Read the model definition and answer for the solid it produces. Units are mm, in the model's axes. A direction names the side the tool comes from. Coordinates: 2 decimals unless noted, no trailing zeros. Order: outer loops, then holes, each group sorted by start corner. A loop starts at its lowest first (then second) coordinate and runs counter-clockwise, first axis right, second up.
from build123d import *

# Parameters (mm, degrees)
BOSS_EXTRUDE1_DEPTH = 4.7625
SKETCH1_3_W         = 6.35
SKETCH1_3_H         = 9.525
SKETCH1_3_H_2       = 6.35
BOSS_EXTRUDE2_DEPTH = 28.73375
SKETCH2_W           = 12.7
SKETCH2_H           = 6.35
SKETCH2_R           = 2.15265
BOSS_EXTRUDE3_DEPTH = 3.175
FILLET11_R          = 3.81


with BuildPart() as part:
    # Sketch1 → Boss-Extrude1 (new body)
    with BuildSketch(Plane(origin=(0, 0, 0), x_dir=(1, 0, 0), z_dir=(0, 1, 0))):
        Polygon((-49.68875, 4.7625), (-49.68875, -4.7625), (49.68875, -4.7625), (49.68875, 4.7625), (-12.7, 4.7625), (-12.7, 12.303125), (-19.05, 12.303125), (-19.05, 4.7625), align=None)
    extrude(amount=BOSS_EXTRUDE1_DEPTH)

    # Sketch1_3 → Boss-Extrude2 (add)
    with BuildSketch(Plane(origin=(0, 0, 0), x_dir=(1, 0, 0), z_dir=(0, 1, 0))):
        with Locations((-46.51375, 0)):
            Rectangle(SKETCH1_3_W, SKETCH1_3_H)
        with Locations((46.51375, 0)):
            Rectangle(SKETCH1_3_W, SKETCH1_3_H)
        with Locations((-15.875, 9.128125)):
            Rectangle(SKETCH1_3_W, SKETCH1_3_H_2)
    extrude(amount=-BOSS_EXTRUDE2_DEPTH)

    # Mirror1: part across plane


with BuildPart() as part_1:
    add(part.part)
    add(part.part.mirror(Plane(origin=(0, 0, 0), x_dir=(0, 0, 1), z_dir=(1, 0, 0))))

    # Sketch2 → Boss-Extrude3 (add)
    with BuildSketch(Plane.XZ.offset(28.73375)):
        with Locations((-6.35, -9.128125)):
            Rectangle(SKETCH2_W, SKETCH2_H)
        with BuildLine():
            Line((-49.68875, 4.7625), (-49.68875, -13.814359467))
            ThreePointArc((-49.68875, -13.814359467), (-44.838220371, -15.559917245), (-40.842233144, -12.303125))
            Line((-40.842233144, -12.303125), (-15.875, -12.303125))
            Line((-15.875, -12.303125), (-15.875, -5.953125))
            Line((-15.875, -5.953125), (-43.33875, -5.953125))
            Line((-43.33875, -5.953125), (-43.33875, 4.7625))
            Line((-43.33875, 4.7625), (-49.68875, 4.7625))
        make_face()
        with Locations(Location((-45.72, -10.398125, 0), (0, 0, 270))):
            Circle(SKETCH2_R, mode=Mode.SUBTRACT)
    boss_extrude3 = extrude(amount=-BOSS_EXTRUDE3_DEPTH)

    # Mirror3: Boss-Extrude3 across plane
    add(boss_extrude3.mirror(Plane(origin=(0, 0, 0), x_dir=(0, 0, 1), z_dir=(1, 0, 0))))

    # Fillet11
    fillet11_edges = [part_1.edges().sort_by_distance(p)[0] for p in [
        (0, 4.7625, 4.7625),
        (-49.68875, -11.985625, 4.7625),
        (49.68875, -11.985625, 4.7625),
    ]]
    fillet(fillet11_edges, radius=FILLET11_R)


solid = part_1.part
Q1. The part is cut by section C-C, the plane z = -3.5. Determine the outline of the cut face in (x, y), then the cut area to 3 significant figures.
Q2. The part is cut by section B-B, the plane x = 39.5. Determine the outline of the cut face in (y, z), then the cut area to 3 significant figures.
Q3. The part is cut by section A-A, the plane y = -13. Determine the outline of the cut face in (x, z), then the cut area to 3 significant figures.
Q4. Each of these flat-tipped pins is pushed along its axis until it touches: P1, Ø1.4, axis at x = 6.5, y = 3, coming from the -Z side; P2, Ø4, axis at y = -16, z = -10, coming from the +X side; P3, Ø1, axis at x = -33, z = 2, coming from the -Y side; P4, Ø12, axis at x = 35.5, z = -7.5, coming from the +Y side. Where does it stop, or does it pass through?
Q5. Determine the mould class of faces 1 (the cylindrical face through (-48.6, -11.75, 3.62)), 2 (the cylindrical face through (47.82, -27.17, -9.93)), 3 (the flat face through (0, 2, -4.762)), 4 (the cylindrical face through (0.696, 3.617, 3.676)) for opening direction X: +X half, -X half, draft (parallel to the pull), parting line (faces both ways), or undercut.
Q6. Which of the six approach directions +Z, -Z, +X, -X, +Y, -Y give full straight-line access (tool end or side, diameter ignored) to faces 5 (the flat face through (12.7, -11, -8)), 6 (the flat face through (0, -26, -5.953)), 7 (the flat face through (-35, -25.559, -9)), 8 (the flat face through (35, -25.559, -9))?
Q7. The part is cut by section D-D, the plane z = -10.5. Determine the outline of the cut face in (x, y).
Q8. Straight lines are drawn through the part: L1, parallel to X at y = -19, z = -4; L2, parallel to X at y = -5.5, z = -6; L3, parallel to Z at x = 45.72, y = -27.55. For each, find the intervals that lie inside material, in ascending order.
Computed values:
1. outline: (-49.69, -28.73) - (-43.34, -28.73) - (-43.34, 0) - (43.34, 0) - (43.34, -28.73) - (49.69, -28.73) - (49.69, 4.76) - (-49.69, 4.76) - close
1. area: 838 mm2
2. outline: (-28.73, -12.3) - (-25.56, -12.3) - (-25.56, -5.95) - (-28.73, -5.95) - close; (0, -4.76) - (4.76, -4.76) - (4.76, 0.95) arc R3.81 ccw to (0.95, 4.76) - (0, 4.76) - close
2. area: 62.4 mm2
3. outline: (-49.69, -4.76) - (-43.34, -4.76) - (-43.34, 4.76) - (-45.88, 4.76) arc R3.81 ccw to (-49.69, 0.95) - close; (-19.05, -12.3) - (-12.7, -12.3) - (-12.7, -5.95) - (-19.05, -5.95) - close; (12.7, -12.3) - (19.05, -12.3) - (19.05, -5.95) - (12.7, -5.95) - close; (43.34, -4.76) - (49.69, -4.76) - (49.69, 0.95) arc R3.81 ccw to (45.88, 4.76) - (43.34, 4.76) - close
3. area: 195 mm2
4. P1: stops at z = -4.76
4. P2: stops at x = 19.05
4. P3: stops at y = 0
4. P4: stops at y = 4.76
5. face 1: -X half
5. face 2: undercut
5. face 3: undercut
5. face 4: draft
6. face 5: -Z, +Y
6. face 6: +Z, -Y
6. face 7: -Z, -X, +Y
6. face 8: -Z, +X, +Y
7. outline: (-49.69, -28.73) - (-47.87, -28.73) - (-47.87, -25.56) - (-49.69, -25.56) - close; (-43.57, -28.73) - (43.57, -28.73) - (43.57, -25.56) - (19.05, -25.56) - (19.05, 4.76) - (12.7, 4.76) - (12.7, -25.56) - (-12.7, -25.56) - (-12.7, 4.76) - (-19.05, 4.76) - (-19.05, -25.56) - (-43.57, -25.56) - close; (47.87, -28.73) - (49.69, -28.73) - (49.69, -25.56) - (47.87, -25.56) - close
8. L1: x = -49.69 to -43.34, 43.34 to 49.69
8. L2: x = -19.05 to -12.7, 12.7 to 19.05
8. L3: z = -15.63 to -12.55, -8.25 to 4.76
